```python
from build123d import *

# Parameters (mm, degrees)
SKETCH_W        = 23
SKETCH_H        = 12
PAD_DEPTH       = 1
SKETCH001_W     = 4
SKETCH001_H     = 4
SKETCH001_W_2   = 9
SKETCH001_W_3   = 1.8
SKETCH001_H_2   = 2.119738
SKETCH001_W_4   = 1.7
SKETCH001_H_3   = 1.880262
SKETCH001_H_4   = 2.108956
SKETCH001_W_5   = 1.95
SKETCH001_H_5   = 1.880263
SKETCH001_H_6   = 2.119737
POCKET_DEPTH    = 5
SKETCH002_W     = 16
SKETCH002_H     = 12
POCKET001_DEPTH = 5
SKETCH003_W     = 0.92929
SKETCH003_H     = 12
POCKET002_DEPTH = 5


with BuildPart() as part:
    # Sketch → Pad (new body)
    with BuildSketch(Plane.XZ):
        with Locations((0.224666, -4.175566)):
            Rectangle(SKETCH_W, SKETCH_H)
    extrude(amount=PAD_DEPTH)

    # Sketch001 (on Face6 of Pad) → Pocket (cut)
    with BuildSketch(Plane.XZ.offset(1)):
        with Locations((-7.275334, -6.675566)):
            Rectangle(SKETCH001_W, SKETCH001_H)
        with Locations((7.724666, -6.675566)):
            Rectangle(SKETCH001_W, SKETCH001_H)
        with Locations((0.224666, -6.675566)):
            Rectangle(SKETCH001_W_2, SKETCH001_H)
        with Locations((-8.375334, -0.735435)):
            Rectangle(SKETCH001_W_3, SKETCH001_H_2)
        with Locations((-6.125334, -0.735435)):
            Rectangle(SKETCH001_W_4, SKETCH001_H_2)
        with Locations((-8.375334, -3.235435)):
            Rectangle(SKETCH001_W_3, SKETCH001_H_3)
        with Locations((-6.125334, -3.235435)):
            Rectangle(SKETCH001_W_4, SKETCH001_H_3)
        with Locations((-3.375334, -0.730044)):
            Rectangle(SKETCH001_W_3, SKETCH001_H_4)
        with Locations((-1.000334, -0.730044)):
            Rectangle(SKETCH001_W_5, SKETCH001_H_4)
        with Locations((-3.375334, -3.224654)):
            Rectangle(SKETCH001_W_3, SKETCH001_H_5)
        with Locations((-1.000334, -3.224654)):
            Rectangle(SKETCH001_W_5, SKETCH001_H_5)
        with Locations((1.374666, -0.730044)):
            Rectangle(SKETCH001_W_3, SKETCH001_H_4)
        with Locations((3.674666, -0.724653)):
            Rectangle(SKETCH001_W_3, SKETCH001_H_6)
        with Locations((1.374666, -3.224654)):
            Rectangle(SKETCH001_W_3, SKETCH001_H_5)
        with Locations((3.749666, -3.224654)):
            Rectangle(SKETCH001_W_5, SKETCH001_H_5)
        with Locations((6.624666, -0.732224)):
            Rectangle(SKETCH001_W_3, SKETCH001_H_2)
        with Locations((8.874666, -0.732224)):
            Rectangle(SKETCH001_W_4, SKETCH001_H_2)
        with Locations((6.624666, -3.232224)):
            Rectangle(SKETCH001_W_3, SKETCH001_H_3)
        with Locations((8.874666, -3.232224)):
            Rectangle(SKETCH001_W_4, SKETCH001_H_3)
    extrude(amount=-POCKET_DEPTH, mode=Mode.SUBTRACT)

    # Sketch002 (on Face5 of Pocket) → Pocket001 (cut)
    with BuildSketch(Plane.XZ.offset(1)):
        with Locations((3.724666, -4.175566)):
            Rectangle(SKETCH002_W, SKETCH002_H)
    extrude(amount=-POCKET001_DEPTH, mode=Mode.SUBTRACT)

    # Sketch003 (on Face4 of Pocket001) → Pocket002 (cut)
    with BuildSketch(Plane.XZ.offset(1)):
        with Locations((-10.810689, -4.175566)):
            Rectangle(SKETCH003_W, SKETCH003_H)
    extrude(amount=-POCKET002_DEPTH, mode=Mode.SUBTRACT)


solid = part.part
```
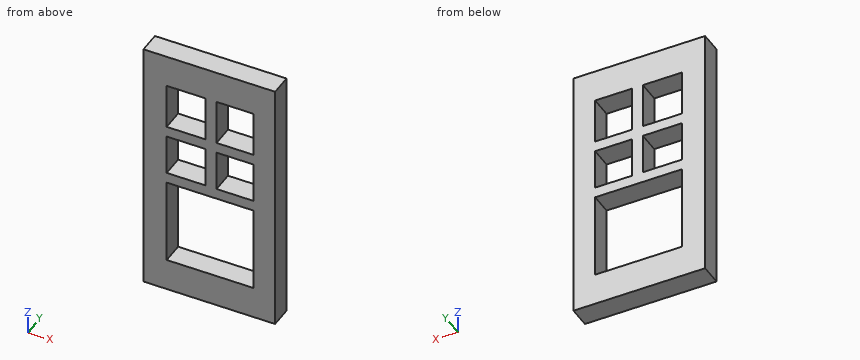
Here's how the part is built. I have some questions about the finished solid (model axes, mm). Round coordinates to 2 decimals unless told otherwise and drop trailing zeros. Order: outer loops, then holes, each group sorted by start corner. A loop starts at its lowest first (then second) coordinate and runs counter-clockwise, first axis right, second up. Notation, with made-up numbers: M 29,50 L 78,50 A15 cw 78,66 Z; hole C -20.5,-8.75 d11. An arc over 180 degrees is marked long. One line per question, with ' | ' between items.
1) I want a section at D-D, the plane x = -6. Write out the boundary of the cut face in (y, z).
Working result:
outline: M -1,-10.18 L 0,-10.18 L 0,-8.68 L -1,-8.68 Z; M -1,-4.68 L 0,-4.68 L 0,-4.18 L -1,-4.18 Z; M -1,-2.3 L 0,-2.3 L 0,-1.8 L -1,-1.8 Z; M -1,0.32 L 0,0.32 L 0,1.82 L -1,1.82 Z
2) I want a section at B-B, the plane y = -0.7. Write out the boundary of the cut face in (x, z), then the cut area to 3 significant figures.
Working result:
outline: M -10.35,-10.18 L -4.28,-10.18 L -4.28,1.82 L -10.35,1.82 Z; hole M -9.28,-8.68 L -5.28,-8.68 L -5.28,-4.68 L -9.28,-4.68 Z; hole M -9.28,-4.18 L -7.48,-4.18 L -7.48,-2.3 L -9.28,-2.3 Z; hole M -9.28,-1.8 L -7.48,-1.8 L -7.48,0.32 L -9.28,0.32 Z; hole M -6.98,-4.18 L -5.28,-4.18 L -5.28,-2.3 L -6.98,-2.3 Z; hole M -6.98,-1.8 L -5.28,-1.8 L -5.28,0.32 L -6.98,0.32 Z | area: 42.8 mm²
3) I want a section at A-A, the plane z = -6.5. Write out the boundary of the cut face in (x, y).
Working result:
outline: M -10.35,-1 L -9.28,-1 L -9.28,0 L -10.35,0 Z; M -5.28,-1 L -4.28,-1 L -4.28,0 L -5.28,0 Z
4) I need wall thicknesses on line 1 along X through (y, z) = (-0.15, -3.5); line 2 along Z through (x, y) = (-6, -0.15); line 3 along X through (y, z) = (-0.15, -5.25). Which ranges of each line are inside material? Lowest first, please.
Working result:
line 1: -10.35 to -9.28, -7.48 to -6.98, -5.28 to -4.28 | line 2: -10.18 to -8.68, -4.68 to -4.18, -2.3 to -1.8, 0.32 to 1.82 | line 3: -10.35 to -9.28, -5.28 to -4.28
5) For pin 1 Ø1 at (x, z) = (-6.5, -6.5) entering from -Y, with a flat end and sliding along its axis, tell me the tip position at first contact or that it passes through.
Working result:
pin 1: through
6) I want a section at C-C, the plane z = -3.5. Write out the boundary of the cut face in (x, y).
Working result:
outline: M -10.35,-1 L -9.28,-1 L -9.28,0 L -10.35,0 Z; M -7.48,-1 L -6.98,-1 L -6.98,0 L -7.48,0 Z; M -5.28,-1 L -4.28,-1 L -4.28,0 L -5.28,0 Z
